Here's how the part is built. I have some questions about the finished solid (model axes, mm). Face numbers are marked on the shaded views. A direction names the side the tool comes from. Round coordinates to 2 decimals unless told otherwise and drop trailing zeros. Write each loop counter-clockwise with the first axis right and the second up, starting at its lowest first coordinate (ties: lowest second). Pieces come first, ordered by that corner, then holes. Notation, with made-up numbers: (36.25, 82) -> (73.25, 82) arc R31 ccw to (73.25, 117) -> close; hole circle Ø4 at (67, 49). An arc over 180 degrees is marked (long way). Answer in a Markdown table with one row per item.
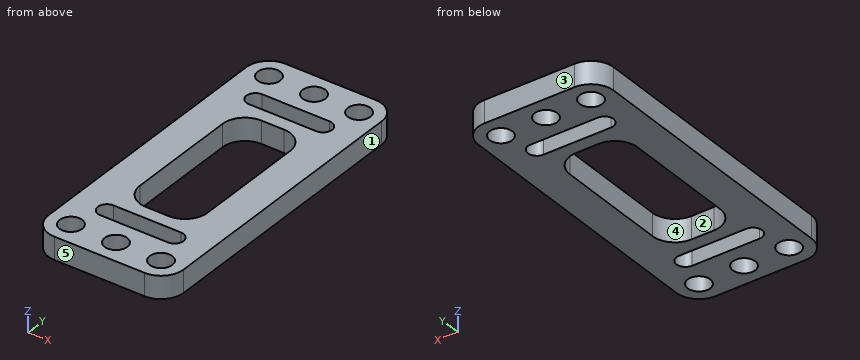
from build123d import *

# Parameters (mm, degrees)
SKETCH1_W           = 30
SKETCH1_H           = 70
SKETCH1_R           = 2.5
BOSS_EXTRUDE1_DEPTH = 5
FILLET1_R           = 5
SKETCH2_W           = 15
SKETCH2_H           = 35
CUT_EXTRUDE1_DEPTH  = 39.405728739
CUT_EXTRUDE2_DEPTH  = 39.405728739
FILLET2_R           = 5


with BuildPart() as part:
    # Sketch1 → Boss-Extrude1 (new body)
    with BuildSketch(Plane.XY):
        Rectangle(SKETCH1_W, SKETCH1_H)
        with Locations((0, 30)):
            Circle(SKETCH1_R, mode=Mode.SUBTRACT)
        with Locations((10, 30)):
            Circle(SKETCH1_R, mode=Mode.SUBTRACT)
        with Locations(Location((-10, 30, 0), (0, 0, 180))):
            Circle(SKETCH1_R, mode=Mode.SUBTRACT)
        with Locations(Location((10, -30, 0), (0, 0, 180))):
            Circle(SKETCH1_R, mode=Mode.SUBTRACT)
        with Locations(Location((0, -30, 0), (0, 0, 180))):
            Circle(SKETCH1_R, mode=Mode.SUBTRACT)
        with Locations((-10, -30)):
            Circle(SKETCH1_R, mode=Mode.SUBTRACT)
    extrude(amount=BOSS_EXTRUDE1_DEPTH)

    # Fillet1
    fillet1_edges = [part.edges().sort_by_distance(p)[0] for p in [
        (15, -35, 2.5),
        (-15, -35, 2.5),
        (-15, 35, 2.5),
        (15, 35, 2.5),
    ]]
    fillet(fillet1_edges, radius=FILLET1_R)

    # Sketch2 → Cut-Extrude1 (cut, through all)
    with BuildSketch(Plane.XY.offset(5)):
        Rectangle(SKETCH2_W, SKETCH2_H)
    extrude(amount=-CUT_EXTRUDE1_DEPTH, mode=Mode.SUBTRACT)

    # Sketch3 → Cut-Extrude2 (cut, through all)
    with BuildSketch(Plane.XY.offset(5)):
        with BuildLine():
            Line((-7.5, 24.5), (7.5, 24.5))
            ThreePointArc((7.5, 24.5), (9.5, 22.5), (7.5, 20.5))
            Line((7.5, 20.5), (-7.5, 20.5))
            ThreePointArc((-7.5, 20.5), (-9.5, 22.5), (-7.5, 24.5))
        make_face()
        with BuildLine():
            Line((-7.5, -24.5), (7.5, -24.5))
            ThreePointArc((7.5, -24.5), (9.5, -22.5), (7.5, -20.5))
            Line((7.5, -20.5), (-7.5, -20.5))
            ThreePointArc((-7.5, -20.5), (-9.5, -22.5), (-7.5, -24.5))
        make_face()
    extrude(amount=-CUT_EXTRUDE2_DEPTH, mode=Mode.SUBTRACT)

    # Fillet2
    fillet2_edges = [part.edges().sort_by_distance(p)[0] for p in [
        (7.5, 17.5, 2.5),
        (7.5, -17.5, 2.5),
        (-7.5, -17.5, 2.5),
        (-7.5, 17.5, 2.5),
    ]]
    fillet(fillet2_edges, radius=FILLET2_R)


solid = part.part
1) I want a section at A-A, the plane z = 2.8. Count the separate pieces of the cut face and the enclosed holes in it, and give its area (3 significant figures).
Response:
| item | result |
|---|---|
| separate pieces | 1 |
| enclosed holes | 9 |
| area | 1,310 mm^2 |
2) For pin 1 (8 mm diameter, centred on x = 0, y = -30, fed in from -Z), with a flat end and sliding along its axis, tell me the tip position at first contact or that it passes through.
Response:
| item | result |
|---|---|
| pin 1 | stops at z = 0 |
3) Which directions (+Z, -Z, +X, -X, +Y, -Y) give clear straight access to the entire face, cutting with the end or side of a thin tool? Please do the marked faces 4 and 5.
Response:
| item | result |
|---|---|
| face 4 | +Z, -Z |
| face 5 | +Z, -Z, +X, -X, -Y |
4) We'd pull the mould along X, two halves only. Please class the marked faces 1, 2 and 3: +X half, -X half, draft (parallel to the pull), parting line (faces both ways), or undercut.
Response:
| item | result |
|---|---|
| face 1 | +X half |
| face 2 | undercut |
| face 3 | draft |
5) I want a section at B-B, the plane y = -22.5. List the corners of the cut face in (x, z) for me, and give its area (3 significant figures).
Response:
| item | result |
|---|---|
| outline | (-15, 0) -> (-9.5, 0) -> (-9.5, 5) -> (-15, 5) -> close; (9.5, 0) -> (15, 0) -> (15, 5) -> (9.5, 5) -> close |
| area | 55.0 mm^2 |
6) I want a section at D-D, the plane x = 11.25. List the corners of the cut face in (y, z) for me, and give its area (3 significant figures).
Response:
| item | result |
|---|---|
| outline | (-34.84, 0) -> (-32.17, 0) -> (-32.17, 5) -> (-34.84, 5) -> close; (-27.83, 0) -> (27.83, 0) -> (27.83, 5) -> (-27.83, 5) -> close; (32.17, 0) -> (34.84, 0) -> (34.84, 5) -> (32.17, 5) -> close |
| area | 305 mm^2 |
7) I want a section at C-C, the plane x = 0. List the corners of the cut face in (y, z) for me, and give its area (3 significant figures).
Response:
| item | result |
|---|---|
| outline | (-35, 0) -> (-32.5, 0) -> (-32.5, 5) -> (-35, 5) -> close; (-27.5, 0) -> (-24.5, 0) -> (-24.5, 5) -> (-27.5, 5) -> close; (-20.5, 0) -> (-17.5, 0) -> (-17.5, 5) -> (-20.5, 5) -> close; (17.5, 0) -> (20.5, 0) -> (20.5, 5) -> (17.5, 5) -> close; (24.5, 0) -> (27.5, 0) -> (27.5, 5) -> (24.5, 5) -> close; (32.5, 0) -> (35, 0) -> (35, 5) -> (32.5, 5) -> close |
| area | 85.0 mm^2 |
8) I need wall thicknesses on line 1 (Y direction, x = -10, z = 1.2); line 2 (Y direction, x = 8.25, z = 1.7); line 3 (Y direction, x = 8.75, z = 1.35). Which ranges of each line are inside material? Lowest first, please. Write a range as [from, to].
Response:
| item | result |
|---|---|
| line 1 | y = [-35, -32.5], [-27.5, 27.5], [32.5, 35] |
| line 2 | y = [-35, -31.79], [-28.21, -24.35], [-20.65, 20.65], [24.35, 28.21], [31.79, 35] |
| line 3 | y = [-35, -32.17], [-27.83, -24.06], [-20.94, 20.94], [24.06, 27.83], [32.17, 35] |
